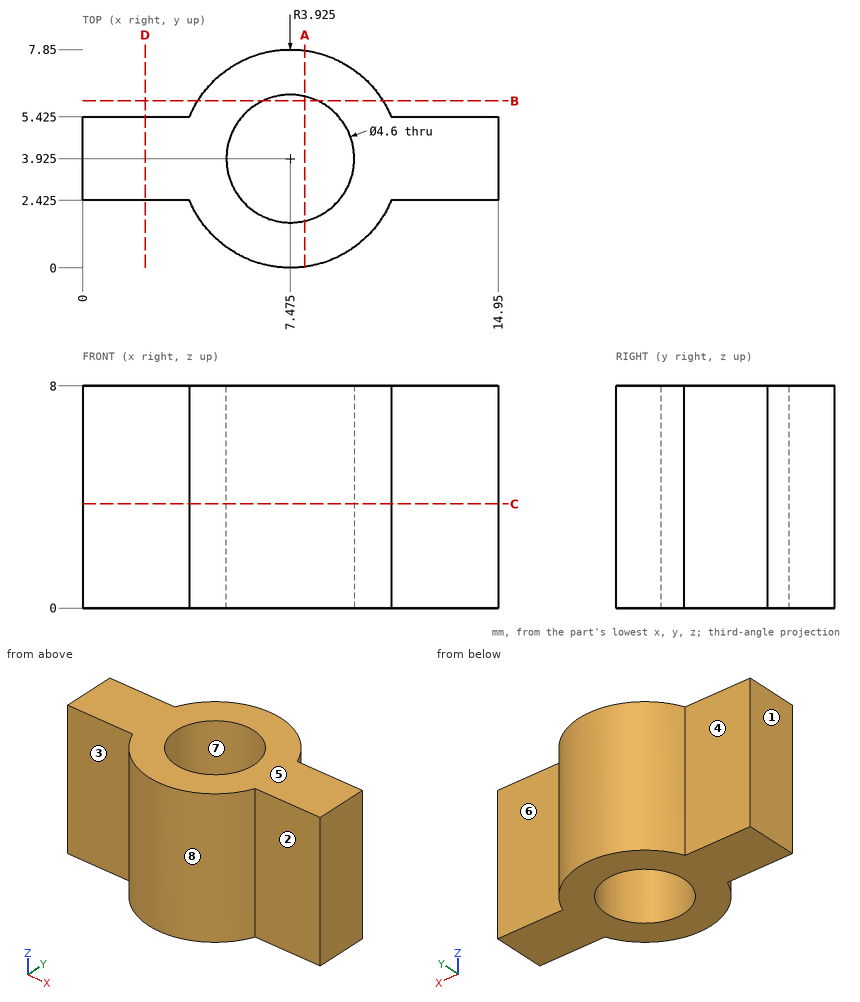
Can you work these out from the drawing? Everything is in mm from the part's minimum corner. A direction names the side the tool comes from. Round coordinates to 2 decimals unless told otherwise and drop trailing zeros. Order: outer loops, then holes, each group sorted by start corner. A loop starts at its lowest first (then second) coordinate and runs counter-clockwise, first axis right, second up.
(1) If we section it at B-B (y = 6): Please give me the cut outline in (x, z), plus the area to 3 significant figures.
Results are:
outline: (4.14, 0) - (6.48, 0) - (6.48, 8) - (4.14, 8) - close; (8.47, 0) - (10.81, 0) - (10.81, 8) - (8.47, 8) - close
area: 37.4 mm2
(2) On a 3-axis mill with a long thin cutter (end or side, diameter ignored), from which of +Z, -Z, +X, -X, +Y, -Y can I reach the whole of each face in a straight line? I mean the marked faces 1, 2, 3, 4 and 5. Say none if no direction works.
Results are:
face 1: +Z, -Z, -X, +Y, -Y
face 2: +Z, -Z, +X, -Y
face 3: +Z, -Z, -X, -Y
face 4: +Z, -Z, -X, +Y
face 5: +Z, +X, -X, +Y, -Y
(3) We'd pull the mould along X, two halves only. Please class the marked faces 6, 7 and 8: +X half, -X half, draft (parallel to the pull), parting line (faces both ways), or undercut.
Results are:
face 6: draft
face 7: undercut
face 8: parting line
(4) I'm going to push flat-ended pins straight in: pin 1 (3 mm diameter, centred on x = 2, z = 3.5, fed in from +Y) (3 decimals); pin 2 (3 mm diameter, centred on x = 9.5, z = 3.5, fed in from +Y); pin 3 (1.9 mm diameter, centred on x = 1, z = 5.5, fed in from -Y) (3 decimals). Where does each tip first touch, or does it pass through?
Results are:
pin 1: stops at y = 5.425
pin 2: stops at y = 7.81
pin 3: stops at y = 2.425
(5) If we section it at D-D (x = 2.25): Please give me the cut outline in (y, z) (3 decimals).
Results are:
outline: (2.425, 0) - (5.425, 0) - (5.425, 8) - (2.425, 8) - close
(6) If I drill on L1, parallel to X at y = 4, z = 5.5; L2, parallel to Y at x = 13, z = 3.5 (3 decimals); L3, parallel to Y at x = 8.5, z = 6.75, over which ranges is the centre line in solid material (lowest first)?
Results are:
L1: x = 0 to 5.18, 9.77 to 14.95
L2: y = 2.425 to 5.425
L3: y = 0.14 to 1.87, 5.98 to 7.71
(7) If we section it at C-C (z = 3.75): Please give me the cut outline in (x, y) (3 decimals).
Results are:
outline: (0, 2.425) - (3.848, 2.425) arc R3.925 ccw to (11.102, 2.425) - (14.95, 2.425) - (14.95, 5.425) - (11.102, 5.425) arc R3.925 ccw to (3.848, 5.425) - (0, 5.425) - close; hole circle Ø4.6 at (7.475, 3.925)
(8) If we section it at A-A (x = 8): Please give me the cut outline in (y, z), plus the area to 3 significant figures.
Results are:
outline: (0.04, 0) - (1.69, 0) - (1.69, 8) - (0.04, 8) - close; (6.16, 0) - (7.81, 0) - (7.81, 8) - (6.16, 8) - close
area: 26.4 mm2
